Check sheet for the modelled part. Datum: model origin and axes. Units: mm. A direction names the side the tool comes from. Coordinates: 2 decimals unless noted, no trailing zeros. Write each loop counter-clockwise with the first axis right and the second up, starting at its lowest first coordinate (ties: lowest second). Pieces come first, ordered by that corner, then holes. Notation, with made-up numbers: (35, 31) -> (41, 31) arc R21 cw to (41, 45) -> close; hole circle Ø2 at (17.25, 52.5). An arc over 180 degrees is marked (long way). One line per item, written item: value. Start each with the question number.
1) Sectioned sample at D-D on z = -9.75. Enter the section's corners in (x, y), plus the area to 3 significant figures.
2) Gauge pin test, flat ends, axial feed: P1, Ø5, axis at x = 1, y = 1, coming from the +Z side; P2, Ø3, axis at x = 7, y = -7, coming from the -Z side; P3, Ø10, axis at x = 6.5, z = -17.5, coming from the -Y side; P4, Ø3, axis at y = 4.5, z = -4.5, coming from the +X side. Record the tip position at first contact, or that the pin passes through.
3) Scan lines: line 1 along Z through (x, y) = (-1.75, 8); line 2 along Z through (x, y) = (6.5, -5.75); line 3 along X through (y, z) = (-2.5, -10.5). Record each from-to range of solid material in increasing order. Write a range as [from, to].
4) Sectioned sample at C-C on z = -21.25. Enter the section's corners in (x, y).
5) Set-up check for faces 1 (the flat face through (0, 0, 0)), 2 (the flat face through (-8, 3, -19.4)), 3 (the cylindrical face through (8.13, -2.56, -2.46)): record each of +Z, -Z, +X, -X, +Y, -Y from which the full face is reachable in a straight line by a thin tool's end or side.
6) Sectioned sample at A-A on y = 0. Enter the section's corners in (x, z) (3 decimals), plus the area to 3 significant figures.
```python
from build123d import *


with BuildPart() as part:
    # Croquis1 → Revolución1 (revolve)
    with BuildSketch(Plane(origin=(0, 0, 0), x_dir=(0, 0, -1), z_dir=(1, 0, 0)), mode=Mode.PRIVATE) as revoluci_n1_sk:
        Polygon((0, 0), (27, 0), (27, 7.9883), (19.4, 7.9883), (19.4, 8.75), (8.55, 8.75), (8.55, 9.525), (5, 9.525), (5, 8.525), (0, 8.525), align=None)
    revolve(revoluci_n1_sk.sketch.rotate(Axis((0, 0, 0), (0, 0, -1)), 90), axis=Axis((0, 0, 0), (0, 0, -1)))


solid = part.part
```
Answers:
1. outline: circle Ø17.5 at (0, 0)
1. area: 241 mm2
2. P1: stops at z = 0
2. P2: stops at z = -19.4
2. P3: stops at y = -8.62
2. P4: stops at x = 9.01
3. line 1: z = [-19.4, 0]
3. line 2: z = [-19.4, -5]
3. line 3: x = [-8.39, 8.39]
4. outline: circle Ø15.98 at (0, 0)
5. face 1: +Z, +X, -X, +Y, -Y
5. face 2: -Z
5. face 3: +Z
6. outline: (-9.525, -8.55) -> (-8.75, -8.55) -> (-8.75, -19.4) -> (-7.988, -19.4) -> (-7.988, -27) -> (7.988, -27) -> (7.988, -19.4) -> (8.75, -19.4) -> (8.75, -8.55) -> (9.525, -8.55) -> (9.525, -5) -> (8.525, -5) -> (8.525, 0) -> (-8.525, 0) -> (-8.525, -5) -> (-9.525, -5) -> close
6. area: 464 mm2
